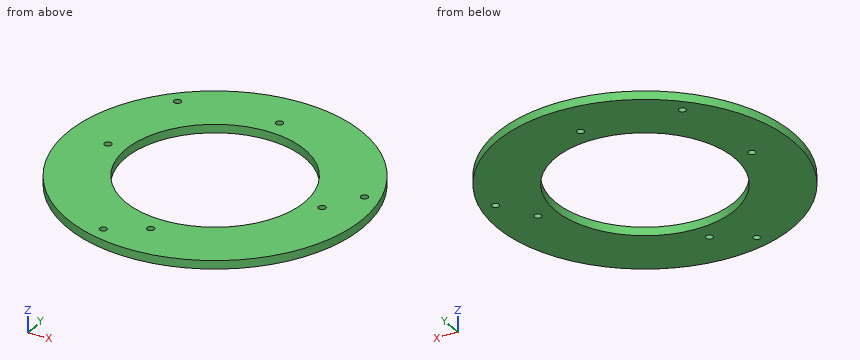
```python
from build123d import *

# Parameters (mm, degrees)
F0_R     = 98.425
F0_R_2   = 2.413
F0_R_3   = 59.69
F1_DEPTH = 5.588


with BuildPart() as f1:
    # F0 (on Top) → F1 (new body)
    with BuildSketch(Plane.XY):
        Circle(F0_R)
        with Locations((-23.009013, -85.870806)):
            Circle(F0_R_2, mode=Mode.SUBTRACT)
        with Locations((0, -71.4629)):
            Circle(F0_R_2, mode=Mode.SUBTRACT)
        with Locations((-71.4629, 0)):
            Circle(F0_R_2, mode=Mode.SUBTRACT)
        with Locations((-62.861793, 62.861793)):
            Circle(F0_R_2, mode=Mode.SUBTRACT)
        Circle(F0_R_3, mode=Mode.SUBTRACT)
        with Locations((71.4629, 0)):
            Circle(F0_R_2, mode=Mode.SUBTRACT)
        with Locations((85.870806, 23.009013)):
            Circle(F0_R_2, mode=Mode.SUBTRACT)
        with Locations((0, 71.4629)):
            Circle(F0_R_2, mode=Mode.SUBTRACT)
    extrude(amount=F1_DEPTH)


solid = f1.part
```
Model file for the job. Use its own axes, mm. Give positions to 0.01 mm unless a question says otherwise; leave off trailing zeros. Order: outer loops, then holes, each group sorted by start corner. A loop starts at its lowest first (then second) coordinate and runs counter-clockwise, first axis right, second up.
1) Saw through at D-D, the plane z = 4.15. Count the separate pieces of the cut face and the enclosed holes in it, then the cut area to 3 significant figures.
2) Saw through at A-A, the plane y = 0. Write the cut outline in (x, z) (3 decimals), then the cut area to 3 significant figures.
3) Saw through at C-C, the plane y = -51.5. Write the cut outline in (x, z), then the cut area to 3 significant figures.
4) Wall check: probe 1 along Y at (x, z) = (0, 2.6) (3 decimals); probe 2 along Y at (x, z) = (-0.5, 4.7); probe 3 along Y at (x, z) = (23, 3.55). Give the ranges that are in metal, low to high.
5) Pin check, flat tips, straight feed: pin 1 (3 mm diameter, centred on x = -30.5, y = 61.5, fed in from -Z); pin 2 (4.5 mm diameter, centred on x = -71.46, y = 0, fed in from -Z); pin 3 (3 mm diameter, centred on x = -26.5, z = 1, fed in from +Y); pin 4 (1 mm diameter, centred on y = 18, z = 3, fed in from -X). Stop position of each tip, or through.
Computed:
1. separate pieces: 1
1. enclosed holes: 8
1. area: 19,100 mm2
2. outline: (-98.425, 0) - (-73.876, 0) - (-73.876, 5.588) - (-98.425, 5.588) - close; (-69.05, 0) - (-59.69, 0) - (-59.69, 5.588) - (-69.05, 5.588) - close; (59.69, 0) - (69.05, 0) - (69.05, 5.588) - (59.69, 5.588) - close; (73.876, 0) - (98.425, 0) - (98.425, 5.588) - (73.876, 5.588) - close
2. area: 379 mm2
3. outline: (-83.88, 0) - (-30.18, 0) - (-30.18, 5.59) - (-83.88, 5.59) - close; (30.18, 0) - (83.88, 0) - (83.88, 5.59) - (30.18, 5.59) - close
3. area: 600 mm2
4. probe 1: y = -98.425 to -73.876, -69.05 to -59.69, 59.69 to 69.05, 73.876 to 98.425
4. probe 2: y = -98.42 to -73.82, -69.1 to -59.69, 59.69 to 69.1, 73.82 to 98.42
4. probe 3: y = -95.7 to -55.08, 55.08 to 95.7
5. pin 1: stops at z = 0
5. pin 2: passes through
5. pin 3: stops at y = 95.2
5. pin 4: stops at x = -96.86
